Input: part model. Units: mm. Frame: model coordinates. A direction names the side the tool comes from. Give positions to 0.01 mm unless a question says otherwise; leave off trailing zeros. Loops run counter-clockwise (first coordinate to the right, second up) from the corner with the lowest first, then second, coordinate; pieces in that order, holes last.
from build123d import *

# Parameters (mm, degrees)
F0_W     = 20
F0_H     = 20
F0_R     = 1.5
F0_R_2   = 2
F0_R_3   = 0.5
F0_R_4   = 1
F1_DEPTH = 2
F2_R     = 1
F2_R_2   = 0.5
F2_R_3   = 2
F2_R_4   = 1.5
F3_DEPTH = 10


with BuildPart() as f1:
    # F0 (on Top) → F1 (new body)
    with BuildSketch(Plane.XY):
        with Locations((-10, -10)):
            Rectangle(F0_W, F0_H)
        with Locations((-14, -14)):
            Circle(F0_R, mode=Mode.SUBTRACT)
        with Locations((-6, -14)):
            Circle(F0_R_2, mode=Mode.SUBTRACT)
        with Locations((-14, -6)):
            Circle(F0_R_3, mode=Mode.SUBTRACT)
        with Locations((-6, -6)):
            Circle(F0_R_4, mode=Mode.SUBTRACT)
        with Locations((-14, -6)):
            Circle(F0_R_3)
        with Locations((-6, -6)):
            Circle(F0_R_4)
        with Locations((-6, -14)):
            Circle(F0_R_2)
        with Locations((-14, -14)):
            Circle(F0_R)
    extrude(amount=F1_DEPTH)

    # F2 (on face) → F3 (join)
    with BuildSketch(Plane.XY.offset(2)):
        with Locations((-6, -6)):
            Circle(F2_R)
        with Locations((-14, -6)):
            Circle(F2_R_2)
        with Locations((-6, -14)):
            Circle(F2_R_3)
        with Locations((-14, -14)):
            Circle(F2_R_4)
    extrude(amount=F3_DEPTH)


solid = f1.part
(1) Cut plane B-B (y = -14). Return the cut outline in (x, z).
Values follow:
outline: (-20, 0) - (0, 0) - (0, 2) - (-4, 2) - (-4, 12) - (-8, 12) - (-8, 2) - (-12.5, 2) - (-12.5, 12) - (-15.5, 12) - (-15.5, 2) - (-20, 2) - close
(2) Cut plane A-A (x = -14). Return the cut outline in (y, z).
Values follow:
outline: (-20, 0) - (0, 0) - (0, 2) - (-5.5, 2) - (-5.5, 12) - (-6.5, 12) - (-6.5, 2) - (-12.5, 2) - (-12.5, 12) - (-15.5, 12) - (-15.5, 2) - (-20, 2) - close
(3) Cut plane C-C (z = 9.25). Return the cut outline in (x, y), and give its area (3 significant figures).
Values follow:
outline: circle Ø3 at (-14, -14); circle Ø1 at (-14, -6); circle Ø4 at (-6, -14); circle Ø2 at (-6, -6)
area: 23.6 mm2
(4) Mould query, pull axis Y, two halves, no side actions, for faces 1 (the flat face through (-10, -20, 1)), 2 (the flat face through (-10, 0, 1)), 3 (the flat face through (0, -10, 1)), 4 (the cylindrical face through (-6.737, -5.324, 6.93)). Classes: +Y half, -Y half, draft (parallel to the pull), parting line (faces both ways), or undercut.
Values follow:
face 1: -Y half
face 2: +Y half
face 3: draft
face 4: undercut
(5) Reachability of faces 5 (the flat face through (-10, -10, 0)), 6 (the cylindrical face through (-6, -12, 7)) from +Z, -Z, +X, -X, +Y, -Y: full face, straight path, thin tool, end or side. Return the list, or none.
Values follow:
face 5: -Z, +X, -X, +Y, -Y
face 6: +Z
(6) Ray query, probe 1 along Z at (x, y) = (-9.25, -6.5); probe 2 along X at (y, z) = (-14.5, 4.5); probe 3 along X at (y, z) = (-14.25, 2.5). Return the intervals inside material, ascending.
Values follow:
probe 1: z = 0 to 2
probe 2: x = -15.41 to -12.59, -7.94 to -4.06
probe 3: x = -15.48 to -12.52, -7.98 to -4.02
(7) Pin query (flat end, axial travel): pin 1 Ø6 at (x, y) = (-16.5, -4) entering from -Z; pin 2 Ø4 at (y, z) = (-12.5, 8) entering from +X; pin 3 Ø1 at (y, z) = (-3, 6.5) entering from +X; pin 4 Ø4 at (y, z) = (-11, 8.5) entering from -X. Return the tip coordinate at first contact, or that it passes through.
Values follow:
pin 1: stops at z = 0
pin 2: stops at x = -4
pin 3: passes through
pin 4: stops at x = -15.12
(8) Cut plane D-D (x = -7.75). Return the cut outline in (y, z).
Values follow:
outline: (-20, 0) - (0, 0) - (0, 2) - (-13.03, 2) - (-13.03, 12) - (-14.97, 12) - (-14.97, 2) - (-20, 2) - close
